Autodesk Inventor part; units mm, degrees
ref_plane "YZ Plane" through (0, 0, 0) normal (1, 0, 0) x (0, 1, 0)
ref_plane "XZ Plane" through (0, 0, 0) normal (0, 1, 0) x (-1, 0, 0)
ref_plane "XY Plane" through (0, 0, 0) normal (0, 0, 1) x (1, 0, 0)
sketch "Sketch1" plane through (0, 0, 0) normal (0, 0, 1) x (1, 0, 0)
  line L0 (0, 0) -> (0, 1479.6195)
  line L1 (0, 1479.6195) -> (-166.4399, 1479.6195)
  line L2 (-166.4399, 1479.6195) -> (-200, 0)
  line L3 (-200, 0) -> (0, 0)
  line L4 (0, 430) -> (-5, 430)
  line L5 (-5, 430) -> (-5, 368)
  line L6 (-5, 368) -> (0, 368)
  line L7 (0, 368) -> (0, 430)
  line L8 (-5, 430) -> (-70, 430)
  line L9 (-70, 430) -> (-70, 425)
  line L10 (-70, 425) -> (-5, 425)
  line L11 (-5, 425) -> (-5, 430)
  line L12 (-70, 430) -> (-190.2469, 430) construction
  line L13 (0, 4408.8661) -> (0, 1479.6195)
  line L14 (-166.4399, 1479.6195) -> (-132.8798, 2959.2389)
  line L15 (0, 4408.8661) -> (-100, 4408.8661)
  line L16 (-132.8798, 2959.2389) -> (0, 2959.2389)
  line L17 (-132.8798, 2959.2389) -> (-100, 4408.8661)
  line L18 (-5, 868) -> (0, 868)
  line L19 (-70, 925) -> (-5, 925)
  line L20 (-5, 930) -> (-70, 930)
  line L21 (-70, 930) -> (-70, 925)
  line L22 (-5, 925) -> (-5, 930)
  line L23 (-5, 930) -> (-5, 868)
  line L24 (0, 868) -> (0, 930)
  line L25 (0, 930) -> (-5, 930)
  line L26 (-5, 1368) -> (0, 1368)
  line L27 (-70, 1425) -> (-5, 1425)
  line L28 (-5, 1430) -> (-70, 1430)
  line L29 (-70, 1430) -> (-70, 1425)
  line L30 (-5, 1425) -> (-5, 1430)
  line L31 (-5, 1430) -> (-5, 1368)
  line L32 (0, 1368) -> (0, 1430)
  line L33 (0, 1430) -> (-5, 1430)
  line L34 (-5, 1868) -> (0, 1868)
  line L35 (-70, 1925) -> (-5, 1925)
  line L36 (-5, 1930) -> (-70, 1930)
  line L37 (-70, 1930) -> (-70, 1925)
  line L38 (-5, 1925) -> (-5, 1930)
  line L39 (-5, 1930) -> (-5, 1868)
  line L40 (0, 1868) -> (0, 1930)
  line L41 (0, 1930) -> (-5, 1930)
  line L42 (-5, 2368) -> (0, 2368)
  line L43 (-70, 2425) -> (-5, 2425)
  line L44 (-5, 2430) -> (-70, 2430)
  line L45 (-70, 2430) -> (-70, 2425)
  line L46 (-5, 2425) -> (-5, 2430)
  line L47 (-5, 2430) -> (-5, 2368)
  line L48 (0, 2368) -> (0, 2430)
  line L49 (0, 2430) -> (-5, 2430)
  line L50 (-5, 2868) -> (0, 2868)
  line L51 (-70, 2925) -> (-5, 2925)
  line L52 (-5, 2930) -> (-70, 2930)
  line L53 (-70, 2930) -> (-70, 2925)
  line L54 (-5, 2925) -> (-5, 2930)
  line L55 (-5, 2930) -> (-5, 2868)
  line L56 (0, 2868) -> (0, 2930)
  line L57 (0, 2930) -> (-5, 2930)
  line L58 (-100, 4408.8661) -> (-99.3197, 4438.8584) construction
  line L59 (0, 1629.6195) -> (-163.0377, 1629.6195)
  line L60 (-131.0653, 3039.2389) -> (0, 3039.2389)
  line L61 (-5, 3368) -> (0, 3368)
  line L62 (-70, 3425) -> (-5, 3425)
  line L63 (-5, 3430) -> (-70, 3430)
  line L64 (-70, 3430) -> (-70, 3425)
  line L65 (-5, 3425) -> (-5, 3430)
  line L66 (-5, 3430) -> (-5, 3368)
  line L67 (0, 3368) -> (0, 3430)
  line L68 (0, 3430) -> (-5, 3430)
  line L69 (-5, 3868) -> (0, 3868)
  line L70 (-70, 3925) -> (-5, 3925)
  line L71 (-5, 3930) -> (-70, 3930)
  line L72 (-70, 3930) -> (-70, 3925)
  line L73 (-5, 3925) -> (-5, 3930)
  line L74 (-5, 3930) -> (-5, 3868)
  line L75 (0, 3868) -> (0, 3930)
  line L76 (0, 3930) -> (-5, 3930)
  arc A0 (-140, 0) -> (-198.6395, 59.9846) centre (-200, 0) ccw
  arc A1 (-167.1202, 1449.6272) -> (-165.7596, 1509.6117) centre (-166.4399, 1479.6195) ccw
  arc A2 (-133.5601, 2929.2466) -> (-132.1995, 2989.2312) centre (-132.8798, 2959.2389) ccw
  line L77 (0, 930) -> (-70, 930)
  line L78 (-70, 930) -> (-178.9061, 930) construction
  line L79 (-70, 1430) -> (-167.5654, 1430) construction
  line L80 (-70, 1930) -> (-156.2246, 1930) construction
  line L81 (-70, 2430) -> (-144.8838, 2430) construction
  line L82 (-70, 2930) -> (-133.543, 2930) construction
  line L83 (-70, 3430) -> (-122.2022, 3430) construction
  line L84 (-70, 3930) -> (-110.8614, 3930) construction
  point P0 (0, 430)
  point P1 (-136.4399, 1479.6195)
  dimension "d25" = 430
  dimension "d32" = 1480
  dimension "d33" = 1480
  dimension "d34" = 1450
  dimension "d35" = 100
  dimension "d38" = 500
  dimension "d44" = 30
  dimension "d45" = 150
  dimension "d46" = 80
  dimension "d47" = 200
  dimension "d48" = 5
  dimension "d50" = 62
  dimension "d51" = 60
  dimension "d52" = 30
  dimension "d53" = 478.8661
  dimension "d54" = 30
  dimension "d56" = 190.2469
  dimension "d57" = 178.9061
  dimension "d58" = 167.5654
  dimension "d59" = 156.2246
  dimension "d60" = 144.8838
  dimension "d61" = 133.543
  dimension "d62" = 122.2022
  dimension "d63" = 110.8614
  dimension "d64" = 70
extrude "Plate1" add sketch "Sketch1" along normal blind 4 contours A1 L14 L59 L13 L1 | L14 A2 L16 L13 L57 L52 L53 L51 L55 L50 L49 L44 L45 L43 L47 L42 L41 L36 L37 L35 L39 L34 L59 | A2 L17 L60 L13 L16
sketch "Sketch2" plane through (4, 1479.6195, 0) normal (-1, 0, 0) x (0, -1, 0)
  line L0 (-388.3805, 0) -> (0, 0)
  line L1 (0, 0) -> (0, -60)
  line L2 (0, -60) -> (-388.3805, -60)
  line L3 (-388.3805, -60) -> (-388.3805, 0)
edge flange "Flange1" height 60 angle 90 thickness 4 bend radius 4 thickness toward (-1, 0, 0) relief tear relief width 4 relief depth 2 corner gap 4 corner form 0 edges at (0, 1673.8097, 0) (0, 2149, 0) (0, 2649, 0) (0, 2984.6195, 0) wall of the first edge with corners at (4, 1868, 0) (4, 1479.6195, 0) (4, 1479.6195, 60) (4, 1868, 60)
bend "Bend1"
corner "Corner1"
chamfer "Corner Chamfer1" distance 10 angle 45 3 edges at (-5, 1925, 2) (-5, 2425, 2) (-5, 2925, 2)
equation "\"d5\" = Thickness"
equation "\"d7\" = BendReliefWidth"
equation "\"d8\" = BendReliefDepth"
equation "\"d9\" = MinimumRemnant"
equation "\"d10\" = TransitionRadius"
equation "\"d13\" = BendRadius"
equation "\"d14\" = CornerReliefSize"
equation "\"d15\" = GapSize"
equation "\"d16\" = JacobiRadiusSize"
equation "\"BendRadius\" = Thickness"
equation "\"BendReliefWidth\" = Thickness"
equation "\"BendReliefDepth\" = 0.5 * Thickness"
equation "\"CornerReliefSize\" = 4 * Thickness"
equation "\"MinimumRemnant\" = 2 * Thickness"
equation "\"TransitionRadius\" = BendRadius"
equation "\"JacobiRadiusSize\" = BendRadius"
equation "\"GapSize\" = Thickness"
properties part number "GBK 0201 second rib" material "Steel"
Geometry: final body of the model. Coordinates: model frame, mm. A direction names the side the tool comes from. Round coordinates to 2 decimals unless told otherwise and drop trailing zeros. Order: outer loops, then holes, each group sorted by start corner. A loop starts at its lowest first (then second) coordinate and runs counter-clockwise, first axis right, second up. Notation, with made-up numbers: M 77,53.5 L 120,53.5 A21 cw 120,84.5 Z; hole C 32,-32 d7. An arc over 180 degrees is marked long. One line per item, written item: value.
(1) Cut plane A-A (z = 27.5). Return the cut outline in (x, y), and give its area (3 significant figures).
Result sheet:
outline: M 0,1479.62 L 4,1479.62 L 4,1868 L 0,1868 Z; M 0,1930 L 4,1930 L 4,2368 L 0,2368 Z; M 0,2430 L 4,2430 L 4,2868 L 0,2868 Z; M 0,2930 L 4,2930 L 4,3039.24 L 0,3039.24 Z
area: 5,490 mm2
(2) Pull-direction query (Y, two-part tool) for faces 4 (the cylindrical face through (-145.216, 1500.822, 1.972)), 5 (the flat face through (-16, 2430, 3)), 6 (the flat face through (0, 1677, 34)), 7 (the flat face through (-16, 2930, 3)); classes: pulls with the +Y half, pulls with the -Y half, needs draft (parallel to the pull), parting line crosses it, or undercut.
Result sheet:
face 4: pulls with the -Y half
face 5: undercut
face 6: needs draft
face 7: undercut
(3) Line query: probe 1 along X at (y, z) = (2946, 9). Output: solid intervals per line, ascending. Write a range as [from, to].
Result sheet:
probe 1: [0, 4]
(4) Cut plane D-D (y = 2018). Return the cut outline in (x, z).
Result sheet:
outline: M -154.23,0 L -4,0 A8 ccw 4,8 L 4,60 L 0,60 L 0,8 A4 cw -4,4 L -154.23,4 Z
(5) Cut plane B-B (x = -30). Return the cut outline in (y, z).
Result sheet:
outline: M 1479.62,0 L 1925,0 L 1925,4 L 1479.62,4 Z; M 1930,0 L 2425,0 L 2425,4 L 1930,4 Z; M 2430,0 L 2925,0 L 2925,4 L 2430,4 Z; M 2930,0 L 3039.24,0 L 3039.24,4 L 2930,4 Z
(6) Cut plane C-C (y = 2446.5). Return the cut outline in (x, z), and give its area (3 significant figures).
Result sheet:
outline: M -144.51,0 L -4,0 A8 ccw 4,8 L 4,60 L 0,60 L 0,8 A4 cw -4,4 L -144.51,4 Z
area: 808 mm2
(7) Reachability of faces 1 (the flat face through (0, 2985, 34)), 2 (the flat face through (-16, 1930, 3)), 3 (the flat face through (4, 2652, 34)) from +Z, -Z, +X, -X, +Y, -Y: full face, straight path, thin tool, end or side. Return the list, or none.
Result sheet:
face 1: +Z, -X, +Y, -Y
face 2: +Z, -Z, +X
face 3: +Z, -Z, +X, +Y, -Y
(8) Pin query (flat end, axial travel): P1, Ø4.5, axis at x = -1.5, z = 32.5, coming from the +Y side; P2, Ø2, axis at y = 2428, z = 2.5, coming from the +X side; P3, Ø4.5, axis at y = 2402, z = 1.5, coming from the +X side; P4, Ø3, axis at x = -46.5, y = 2109.5, coming from the +Z side. Return the tip coordinate at first contact, or that it passes through.
Result sheet:
P1: y = 3039.24
P2: x = -70
P3: x = -5
P4: z = 4
